Read the model definition and answer for the solid it produces. Units are mm, in the model's axes. A direction names the side the tool comes from. Coordinates: 2 decimals unless noted, no trailing zeros. Loops run counter-clockwise (first coordinate to the right, second up) from the corner with the lowest first, then second, coordinate; pieces in that order, holes last. Notation, with made-up numbers: (6, 84.5) - (60, 84.5) arc R10 ccw to (60, 93.5) - close; hole circle Ø3 at (-12.5, 49.25). An arc over 180 degrees is marked (long way). One line per question, with ' | ' between items. Start each with the question number.
```python
from build123d import *

# Parameters (mm, degrees)
BOSS_EXTRUDE1_DEPTH                           = 17
BOSS_EXTRUDE2_START                           = -0.5
BOSS_EXTRUDE2_DEPTH                           = 0.5
CBORE_START                                   = -0.5
CBORE_FOR_M3_HEX_SOCKET_HEAD_CAP_SCR_2_R      = 1.8
CBORE_FOR_M3_HEX_SOCKET_HEAD_CAP_SCREW1_DEPTH = 17.5
CBORE_START_2                                 = 13.6
CBORE_FOR_M3_HEX_SOCKET_HEAD_CAP_SCR_3_O_R    = 3.25
CBORE_FOR_M3_HEX_SOCKET_HEAD_CAP_SCR_3_O_R_2  = 1.8
CBORE_FOR_M3_HEX_SOCKET_HEAD_CAP_SCR_3_DEPTH  = 3.4
F_2_5MM_CHAMFER1_SIZE                         = 2.5
F_0_5MM_CHAMFER2_SIZE                         = 0.5


# Read off the part's stored shape, not the designer's step: CBORE for M3 Hex Socket Head Cap Screw1
with BuildPart() as part:
    # Sketch1 → Boss-Extrude1 (new body)
    with BuildSketch(Plane(origin=(0, 0, 0), x_dir=(0, 0, -1), z_dir=(1, 0, 0))):
        with BuildLine():
            ThreePointArc((-17, 0), (0, 17), (17, 0))
            Line((17, 0), (35, 0))
            ThreePointArc((35, 0), (0, 35), (-35, 0))
            Line((-35, 0), (-17, 0))
        make_face()
        with BuildLine():
            Line((35, 0), (17, 0))
            ThreePointArc((17, 0), (0, -17), (-17, 0))
            Line((-17, 0), (-35, 0))
            ThreePointArc((-35, 0), (0, -35), (35, 0))
        make_face()
        with BuildLine():
            ThreePointArc((-5.5, 0), (0, 5.5), (5.5, 0))
            Line((5.5, 0), (17, 0))
            ThreePointArc((17, 0), (0, 17), (-17, 0))
            Line((-17, 0), (-5.5, 0))
        make_face()
        with BuildLine():
            Line((17, 0), (5.5, 0))
            ThreePointArc((5.5, 0), (0, -5.5), (-5.5, 0))
            Line((-5.5, 0), (-17, 0))
            ThreePointArc((-17, 0), (0, -17), (17, 0))
        make_face()
        with BuildLine():
            Line((35, -70), (35, 0))
            ThreePointArc((35, 0), (0, -35), (-35, 0))
            Line((-35, 0), (-35, -70))
            Line((-35, -70), (35, -70))
        make_face()
    extrude(amount=BOSS_EXTRUDE1_DEPTH)

    # Sketch1<4> → Boss-Extrude2 (add)
    with BuildSketch(Plane(origin=(0, 0, 0), x_dir=(0, 0, -1), z_dir=(1, 0, 0)).offset(BOSS_EXTRUDE2_START)):
        with BuildLine():
            ThreePointArc((-5.5, 0), (0, 5.5), (5.5, 0))
            Line((5.5, 0), (17, 0))
            ThreePointArc((17, 0), (0, 17), (-17, 0))
            Line((-17, 0), (-5.5, 0))
        make_face()
        with BuildLine():
            Line((17, 0), (5.5, 0))
            ThreePointArc((5.5, 0), (0, -5.5), (-5.5, 0))
            Line((-5.5, 0), (-17, 0))
            ThreePointArc((-17, 0), (0, -17), (17, 0))
        make_face()
    extrude(amount=BOSS_EXTRUDE2_DEPTH)

    # CBORE for M3 Hex Socket Head Cap Scr 2 → CBORE for M3 Hex Socket Head Cap Screw1 (cut)
    with BuildSketch(Plane.YZ.offset(CBORE_START)):
        with Locations((-63, -25)):
            Circle(CBORE_FOR_M3_HEX_SOCKET_HEAD_CAP_SCR_2_R)
        with Locations((-43, 25)):
            Circle(CBORE_FOR_M3_HEX_SOCKET_HEAD_CAP_SCR_2_R)
        with Locations((-63, 25)):
            Circle(CBORE_FOR_M3_HEX_SOCKET_HEAD_CAP_SCR_2_R)
        with Locations((-43, -25)):
            Circle(CBORE_FOR_M3_HEX_SOCKET_HEAD_CAP_SCR_2_R)
        with Locations((-53, 0)):
            Circle(CBORE_FOR_M3_HEX_SOCKET_HEAD_CAP_SCR_2_R)
        with Locations((7.071067812, 7.071067812)):
            Circle(CBORE_FOR_M3_HEX_SOCKET_HEAD_CAP_SCR_2_R)
        with Locations((-7.071067812, 7.071067812)):
            Circle(CBORE_FOR_M3_HEX_SOCKET_HEAD_CAP_SCR_2_R)
        with Locations((-7.071067812, -7.071067812)):
            Circle(CBORE_FOR_M3_HEX_SOCKET_HEAD_CAP_SCR_2_R)
        with Locations((7.071067812, -7.071067812)):
            Circle(CBORE_FOR_M3_HEX_SOCKET_HEAD_CAP_SCR_2_R)
    extrude(amount=CBORE_FOR_M3_HEX_SOCKET_HEAD_CAP_SCREW1_DEPTH, mode=Mode.SUBTRACT)

    # CBORE for M3 Hex Socket Head Cap Scr 3 o → CBORE for M3 Hex Socket Head Cap Scr 3 (cut)
    # profile 1 of 9: a face of its own
    with BuildSketch(Plane.YZ.offset(CBORE_START_2)):
        with Locations((-63, -25)):
            Circle(CBORE_FOR_M3_HEX_SOCKET_HEAD_CAP_SCR_3_O_R)
        with Locations((-63, -25)):
            Circle(CBORE_FOR_M3_HEX_SOCKET_HEAD_CAP_SCR_3_O_R_2, mode=Mode.SUBTRACT)
    # profile 2 of 9: a face of its own
    with BuildSketch(Plane.YZ.offset(CBORE_START_2)):
        with Locations((-43, 25)):
            Circle(CBORE_FOR_M3_HEX_SOCKET_HEAD_CAP_SCR_3_O_R)
        with Locations((-43, 25)):
            Circle(CBORE_FOR_M3_HEX_SOCKET_HEAD_CAP_SCR_3_O_R_2, mode=Mode.SUBTRACT)
    # profile 3 of 9: a face of its own
    with BuildSketch(Plane.YZ.offset(CBORE_START_2)):
        with Locations((-63, 25)):
            Circle(CBORE_FOR_M3_HEX_SOCKET_HEAD_CAP_SCR_3_O_R)
        with Locations((-63, 25)):
            Circle(CBORE_FOR_M3_HEX_SOCKET_HEAD_CAP_SCR_3_O_R_2, mode=Mode.SUBTRACT)
    # profile 4 of 9: a face of its own
    with BuildSketch(Plane.YZ.offset(CBORE_START_2)):
        with Locations((-43, -25)):
            Circle(CBORE_FOR_M3_HEX_SOCKET_HEAD_CAP_SCR_3_O_R)
        with Locations((-43, -25)):
            Circle(CBORE_FOR_M3_HEX_SOCKET_HEAD_CAP_SCR_3_O_R_2, mode=Mode.SUBTRACT)
    # profile 5 of 9: a face of its own
    with BuildSketch(Plane.YZ.offset(CBORE_START_2)):
        with Locations((-53, 0)):
            Circle(CBORE_FOR_M3_HEX_SOCKET_HEAD_CAP_SCR_3_O_R)
        with Locations((-53, 0)):
            Circle(CBORE_FOR_M3_HEX_SOCKET_HEAD_CAP_SCR_3_O_R_2, mode=Mode.SUBTRACT)
    # profile 6 of 9: a face of its own
    with BuildSketch(Plane.YZ.offset(CBORE_START_2)):
        with Locations((7.071067812, 7.071067812)):
            Circle(CBORE_FOR_M3_HEX_SOCKET_HEAD_CAP_SCR_3_O_R)
        with Locations((7.071067812, 7.071067812)):
            Circle(CBORE_FOR_M3_HEX_SOCKET_HEAD_CAP_SCR_3_O_R_2, mode=Mode.SUBTRACT)
    # profile 7 of 9: a face of its own
    with BuildSketch(Plane.YZ.offset(CBORE_START_2)):
        with Locations((-7.071067812, 7.071067812)):
            Circle(CBORE_FOR_M3_HEX_SOCKET_HEAD_CAP_SCR_3_O_R)
        with Locations((-7.071067812, 7.071067812)):
            Circle(CBORE_FOR_M3_HEX_SOCKET_HEAD_CAP_SCR_3_O_R_2, mode=Mode.SUBTRACT)
    # profile 8 of 9: a face of its own
    with BuildSketch(Plane.YZ.offset(CBORE_START_2)):
        with Locations((-7.071067812, -7.071067812)):
            Circle(CBORE_FOR_M3_HEX_SOCKET_HEAD_CAP_SCR_3_O_R)
        with Locations((-7.071067812, -7.071067812)):
            Circle(CBORE_FOR_M3_HEX_SOCKET_HEAD_CAP_SCR_3_O_R_2, mode=Mode.SUBTRACT)
    # profile 9 of 9: a face of its own
    with BuildSketch(Plane.YZ.offset(CBORE_START_2)):
        with Locations((7.071067812, -7.071067812)):
            Circle(CBORE_FOR_M3_HEX_SOCKET_HEAD_CAP_SCR_3_O_R)
        with Locations((7.071067812, -7.071067812)):
            Circle(CBORE_FOR_M3_HEX_SOCKET_HEAD_CAP_SCR_3_O_R_2, mode=Mode.SUBTRACT)
    extrude(amount=CBORE_FOR_M3_HEX_SOCKET_HEAD_CAP_SCR_3_DEPTH, mode=Mode.SUBTRACT)

    # 2,5mm Chamfer1
    f_2_5mm_chamfer1_edges = [part.edges().sort_by_distance(p)[0] for p in [
        (17, 35, 0),
        (17, -35, 35),
        (17, -35, -35),
    ]]
    chamfer(f_2_5mm_chamfer1_edges, length=F_2_5MM_CHAMFER1_SIZE)

    # 0,5mm Chamfer2
    f_0_5mm_chamfer2_edges = [part.edges().sort_by_distance(p)[0] for p in [
        (0, -64.8, -25),
        (17, -66.25, -25),
        (0, -44.8, 25),
        (17, -46.25, 25),
        (0, -64.8, 25),
        (17, -66.25, 25),
        (0, -44.8, -25),
        (17, -46.25, -25),
        (17, 0, 5.5),
        (0, -54.8, 0),
        (17, -56.25, 0),
        (17, 3.821067812, 7.071067812),
        (-0.5, 5.271067812, 7.071067812),
        (17, -10.321067812, 7.071067812),
        (-0.5, -8.871067812, 7.071067812),
        (17, -10.321067812, -7.071067812),
        (-0.5, -8.871067812, -7.071067812),
        (17, 3.821067812, -7.071067812),
        (-0.5, 5.271067812, -7.071067812),
    ]]
    chamfer(f_0_5mm_chamfer2_edges, length=F_0_5MM_CHAMFER2_SIZE)


solid = part.part
```
1) The mould has two halves that part along Z. Classify faces 3 (the flat face through (13.6, 8.5, -8.5)), 4 (the flat face through (17, -18, 0)), 5 (the conical face through (16.84, 32.65, -0.72)): released by +Z, released by -Z, zero draft, split by the parting line, or undercut.
2) Find the intervals of material crossed by line 1 along Y through (x, z) = (10.75, 0); line 2 along Z through (x, y) = (11.25, -7); line 3 along Z through (x, y) = (2.75, -42), in increasing order. Write a range as from..to.
3) The part is cut by section B-B on z = 0. Write down the section's boundary in (x, y).
4) Given pin 1 Ø2 at (y, z) = (-7.07, 7.07) entering from -X; pin 2 Ø1.9 at (y, z) = (-8.5, -7.5) entering from +X; pin 3 Ø1 at (x, y) = (12.5, 16.5) entering from -Z; pin 4 Ø6 at (y, z) = (21, 1) entering from -X, each flat-ended and moving along its own axis, determine where each tip first touches the part or whether it passes through.
5) Which of the six approach directions +Z, -Z, +X, -X, +Y, -Y give full straight-line access (tool end or side, diameter ignored) to faces 1 (the flat face through (7, -35, 35)), 2 (the flat face through (13.6, -61.6, 23.6))?
6) The part is cut by section A-A on y = -63. Count the separate pieces of the cut face and the enclosed holes in it, and give its area (3 significant figures).
Answer below:
1) face 3: undercut | face 4: zero draft | face 5: split by the parting line
2) line 1: -70..-54.8, -51.2..-5.5, 5.5..35 | line 2: -35..-8.87, -5.27..5.27, 8.87..35 | line 3: -35..-26.5, -23.5..23.5, 26.5..35
3) outline: (-0.5, -17) - (0, -17) - (0, -50.7) - (0.5, -51.2) - (13.6, -51.2) - (13.6, -49.75) - (16.5, -49.75) - (17, -49.25) - (17, -6) - (16.5, -5.5) - (-0.5, -5.5) - close; (-0.5, 5.5) - (16.5, 5.5) - (17, 6) - (17, 32.5) - (14.5, 35) - (0, 35) - (0, 17) - (-0.5, 17) - close; (0, -70) - (17, -70) - (17, -56.75) - (16.5, -56.25) - (13.6, -56.25) - (13.6, -54.8) - (0.5, -54.8) - (0, -55.3) - close
4) pin 1: through | pin 2: x = 13.6 | pin 3: z = -31.13 | pin 4: x = 0
5) face 1: +Z, +X, -X, +Y, -Y | face 2: +X
6) separate pieces: 3 | enclosed holes: 0 | area: 1,040 mm2
